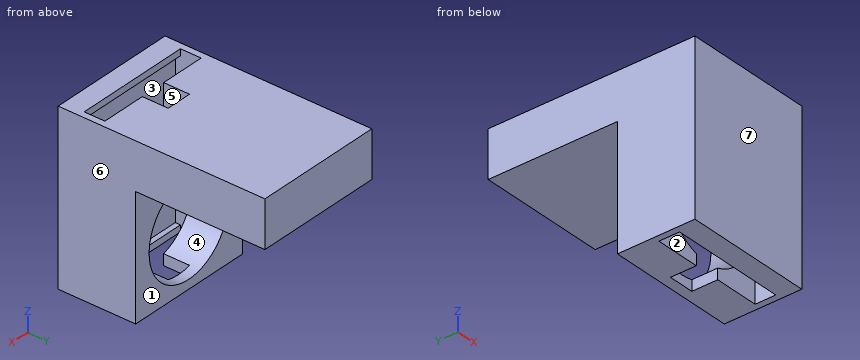
```python
from build123d import *

# Parameters (mm, degrees)
SKETCH1_W           = 50
SKETCH1_H           = 65
BOSS_EXTRUDE1_DEPTH = 30
SKETCH3_W           = 10
SKETCH3_H           = 10
SKETCH3_W_2         = 45
SKETCH3_H_2         = 8
CUT_EXTRUDE4_DEPTH  = 88.321245983
SKETCH4_W           = 60
SKETCH4_H           = 2
CUT_EXTRUDE5_DEPTH  = 45
CUT_EXTRUDE6_REACH  = 89.321
SKETCH5_R           = 18.5
SKETCH6_W           = 50
SKETCH6_H           = 18
BOSS_EXTRUDE2_DEPTH = 50


with BuildPart() as part:
    # Sketch1 → Boss-Extrude1 (new body)
    with BuildSketch(Plane(origin=(0, 0, 0), x_dir=(1, 0, 0), z_dir=(0, 1, 0))):
        with Locations((25, 32.5)):
            Rectangle(SKETCH1_W, SKETCH1_H)
    extrude(amount=BOSS_EXTRUDE1_DEPTH)

    # Sketch3 → Cut-Extrude4 (cut, through all)
    with BuildSketch(Plane.XY):
        with Locations((25, 21)):
            Rectangle(SKETCH3_W, SKETCH3_H)
        with Locations((25, 12)):
            Rectangle(SKETCH3_W_2, SKETCH3_H_2)
    extrude(amount=-CUT_EXTRUDE4_DEPTH, mode=Mode.SUBTRACT)

    # Sketch4 → Cut-Extrude5 (cut)
    with BuildSketch(Plane.ZY.offset(-47.5)):
        with Locations((-32.5, 7)):
            Rectangle(SKETCH4_W, SKETCH4_H)
    extrude(amount=CUT_EXTRUDE5_DEPTH, mode=Mode.SUBTRACT)

    # Cut-Extrude6: up to this face of the body (flat: up to its plane)
    cut_extrude6_end = Plane(part.part.faces().sort_by_distance((11.25, 16, -32.5))[0])
    # Sketch5 → Cut-Extrude6 (cut, up to the picked face)
    with BuildSketch(Plane(origin=(0, 30, 0), x_dir=(1, 0, 0), z_dir=(0, 1, 0)), mode=Mode.PRIVATE) as cut_extrude6_sk1:
        with Locations(Location((25.244510865, 43, 0), (0, 0, 270))):
            Circle(SKETCH5_R)
    cut_extrude6_tool1 = split(extrude(cut_extrude6_sk1.sketch, amount=-CUT_EXTRUDE6_REACH, mode=Mode.PRIVATE), bisect_by=cut_extrude6_end, keep=Keep.BOTH, mode=Mode.PRIVATE)
    add(cut_extrude6_tool1.solids().sort_by(Axis((25.244511, 30, -43), (0, -1, 0)))[0], mode=Mode.SUBTRACT)

    # Sketch6 → Boss-Extrude2 (add)
    with BuildSketch(Plane(origin=(0, 30, 0), x_dir=(1, 0, 0), z_dir=(0, 1, 0))):
        with Locations((25, 9)):
            Rectangle(SKETCH6_W, SKETCH6_H)
    extrude(amount=BOSS_EXTRUDE2_DEPTH)


solid = part.part
```
For this review, take the finished solid that the model builds, in its own axes (mm). Face numbers are marked on the shaded views. A direction names the side the tool comes from. Coordinates: 2 decimals unless noted, no trailing zeros. Loops run counter-clockwise (first coordinate to the right, second up) from the corner with the lowest first, then second, coordinate; pieces in that order, holes last. Notation, with made-up numbers: (-21.75, -5.5) -> (15.25, -5.5) arc R22 cw to (15.25, 12.5) -> close; hole circle Ø1 at (-22, -39.5). An arc over 180 degrees is marked (long way). Return JSON: item names as keys, results as strings. Group by question number.
(1) To check wall thickness, follow L1, parallel to X at y = 21.5, z = -43; L2, parallel to Y at x = 18, z = -20; L3, parallel to Y at x = 19, z = -17. State the ranges of each line that lie inside material, in increasing order.
(2) Consider section B-B, the plane x = 17.5. Give the boundary of the cut face in (y, z).
(3) Consider section A-A, the plane x = 46.5. Give the boundary of the cut face in (y, z), plus the area to 3 significant figures.
(4) For pin 1 Ø5 at (x, z) = (24.5, -21) entering from -Y; pin 2 Ø1.5 at (x, z) = (11.5, -52.5) entering from +Y; pin 3 Ø0.8 at (x, z) = (17.5, -63) entering from +Y; pin 4 Ø6 at (x, y) = (27.5, 48.5) entering from -Z, all flat-tipped, find the tip position at first contact; note any pin that passes through.
(5) Mouldability with a two-part tool opening along X and no side actions: class the marked faces 5, 6 and 7 as pulls with the +X half, pulls with the -X half, needs draft (parallel to the pull), parting line crosses it, or undercut.
(6) Tool access review of the marked faces 1, 2, 3 and 4: name each direction out of +Z, -Z, +X, -X, +Y, -Y from which nothing blocks a thin tool from reaching the whole face with its end or side.
(7) Consider section C-C, the plane z = -43. Give the boundary of the cut face in (x, y).
(8) Consider section D-D, the plane y = 45.5. Give the boundary of the cut face in (x, z).
Results below:
{
 "1": {"L1": "x = 0 to 6.74, 43.74 to 50", "L2": "y = 0 to 6, 16 to 30", "L3": "y = 0 to 6, 16 to 80"},
 "2": {"outline": "(0, -65) -> (8, -65) -> (8, -62.5) -> (6, -62.5) -> (6, -2.5) -> (8, -2.5) -> (8, 0) -> (0, 0) -> close; (16, -65) -> (30, -65) -> (30, -59.8) -> (16, -59.8) -> close; (16, -26.2) -> (30, -26.2) -> (30, -18) -> (80, -18) -> (80, 0) -> (16, 0) -> close"},
 "3": {"outline": "(0, -65) -> (8, -65) -> (8, -62.5) -> (6, -62.5) -> (6, -2.5) -> (8, -2.5) -> (8, 0) -> (0, 0) -> close; (16, -65) -> (30, -65) -> (30, -18) -> (80, -18) -> (80, 0) -> (16, 0) -> close", "area": "2,210 mm2"},
 "4": {"pin 1": "stops at y = 0", "pin 2": "stops at y = 6", "pin 3": "stops at y = 30", "pin 4": "stops at z = -18"},
 "5": {"face 5": "undercut", "face 6": "pulls with the +X half", "face 7": "needs draft"},
 "6": {"face 1": "-Z, +X, -X, +Y", "face 2": "+Z, -Z", "face 3": "none", "face 4": "+Y"},
 "7": {"outline": "(0, 0) -> (50, 0) -> (50, 30) -> (43.74, 30) -> (43.74, 16) -> (47.5, 16) -> (47.5, 6) -> (2.5, 6) -> (2.5, 16) -> (6.74, 16) -> (6.74, 30) -> (0, 30) -> close"},
 "8": {"outline": "(0, -18) -> (50, -18) -> (50, 0) -> (0, 0) -> close"}
}
